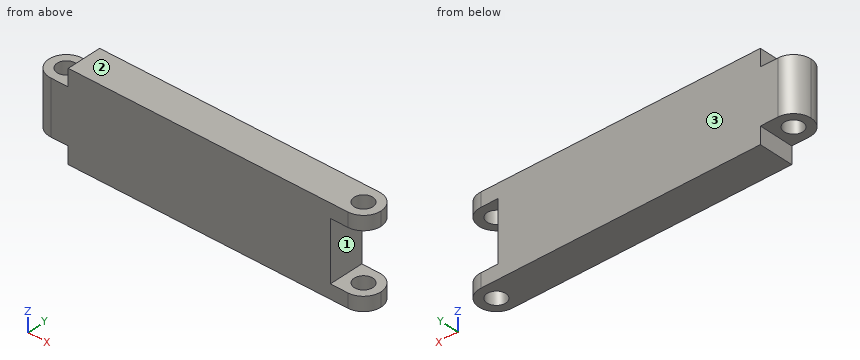
from build123d import *

# Parameters (mm, degrees)
SKETCH_1_W           = 57
SKETCH_1_H           = 15
EXTRUDE_5_DEPTH      = 6
SKETCH_13_W          = 6
SKETCH_13_H          = 10.2
CUT_EXTRUDE_8_DEPTH  = 6
SKETCH_14_R          = 1.6
CUT_EXTRUDE_9_DEPTH  = 17
SKETCH_15_W          = 6
SKETCH_15_H          = 2.4
CUT_EXTRUDE_10_DEPTH = 17
SKETCH_16_R          = 1.6
CUT_EXTRUDE_11_DEPTH = 17
SKETCH_17_W          = 6
SKETCH_17_H          = 6
CUT_EXTRUDE_12_DEPTH = 0.5
SKETCH_18_W          = 6
SKETCH_18_H          = 6
CUT_EXTRUDE_13_DEPTH = 0.5


with BuildPart() as part:
    # 草图1 → 凸台-拉伸5 (new body)
    with BuildSketch(Plane(origin=(0, 0, 0), x_dir=(1, 0, 0), z_dir=(0, 1, 0))):
        with Locations((5.252559727, 3.394197952)):
            Rectangle(SKETCH_1_W, SKETCH_1_H)
    extrude(amount=EXTRUDE_5_DEPTH)

    # 草图13 → 切除-拉伸8 (cut)
    with BuildSketch(Plane(origin=(0, 6, 0), x_dir=(1, 0, 0), z_dir=(0, 1, 0))):
        with Locations((30.752559727, 3.394197952)):
            Rectangle(SKETCH_13_W, SKETCH_13_H)
    extrude(amount=-CUT_EXTRUDE_8_DEPTH, mode=Mode.SUBTRACT)

    # 草图14 → 切除-拉伸9 (cut)
    with BuildSketch(Plane.XY.offset(4.105802048)):
        with Locations((30.752559727, 3)):
            Circle(SKETCH_14_R)
        with BuildLine():
            Line((33.752559727, 6), (30.752559727, 6))
            ThreePointArc((30.752559727, 6), (32.873880071, 5.121320344), (33.752559727, 3))
            Line((33.752559727, 3), (33.752559727, 6))
        make_face()
        with BuildLine():
            Line((33.752559727, 0), (33.752559727, 3))
            ThreePointArc((33.752559727, 3), (32.873880071, 0.878679656), (30.752559727, 0))
            Line((30.752559727, 0), (33.752559727, 0))
        make_face()
    extrude(amount=-CUT_EXTRUDE_9_DEPTH, mode=Mode.SUBTRACT)

    # 草图15 → 切除-拉伸10 (cut)
    with BuildSketch(Plane(origin=(0, 6, 0), x_dir=(1, 0, 0), z_dir=(0, 1, 0))):
        with Locations((-20.247440273, 9.694197952)):
            Rectangle(SKETCH_15_W, SKETCH_15_H)
        with Locations((-20.247440273, -2.905802048)):
            Rectangle(SKETCH_15_W, SKETCH_15_H)
    extrude(amount=-CUT_EXTRUDE_10_DEPTH, mode=Mode.SUBTRACT)

    # 草图16 → 切除-拉伸11 (cut)
    with BuildSketch(Plane.XY.offset(1.705802048)):
        with Locations((-20.247440273, 3)):
            Circle(SKETCH_16_R)
        with BuildLine():
            ThreePointArc((-23.247440273, 3), (-22.368760617, 5.121320344), (-20.247440273, 6))
            Line((-20.247440273, 6), (-23.247440273, 6))
            Line((-23.247440273, 6), (-23.247440273, 3))
        make_face()
        with BuildLine():
            ThreePointArc((-20.247440273, 0), (-22.368760617, 0.878679656), (-23.247440273, 3))
            Line((-23.247440273, 3), (-23.247440273, 0))
            Line((-23.247440273, 0), (-20.247440273, 0))
        make_face()
    extrude(amount=-CUT_EXTRUDE_11_DEPTH, mode=Mode.SUBTRACT)

    # 草图17 → 切除-拉伸12 (cut)
    with BuildSketch(Plane(origin=(0, 0, -8.494197952), x_dir=(-1, 0, 0), z_dir=(0, 0, -1))):
        with Locations((20.247440273, 3)):
            Rectangle(SKETCH_17_W, SKETCH_17_H)
    extrude(amount=-CUT_EXTRUDE_12_DEPTH, mode=Mode.SUBTRACT)

    # 草图18 → 切除-拉伸13 (cut)
    with BuildSketch(Plane.XY.offset(1.705802048)):
        with Locations((-20.247440273, 3)):
            Rectangle(SKETCH_18_W, SKETCH_18_H)
    extrude(amount=-CUT_EXTRUDE_13_DEPTH, mode=Mode.SUBTRACT)


solid = part.part
Can you work these out from the model? Positions are in its coordinate system, mm. Face numbers are marked on the shaded views. Round coordinates to 2 decimals unless told otherwise and drop trailing zeros. Order: outer loops, then holes, each group sorted by start corner. A loop starts at its lowest first (then second) coordinate and runs counter-clockwise, first axis right, second up. Notation, with made-up numbers: (72, 2) -> (131, 2) arc R21 ccw to (131, 40) -> close; hole circle Ø5 at (78.5, 43). An arc over 180 degrees is marked (long way). Write each question's results on one line, items separated by ' | '. Start each with the question number.
Item 1: Thinking about a two-plate mould opening in Z: for the marked faces 1, 2 and 3, which applies, +Z half, -Z half, draft (parallel to the pull), parting line (faces both ways), or undercut?
Item 2: If we section it at B-B, the plane y = 0.5: Write out the boundary of the cut face in (x, z), then the cut area to 3 significant figures.
Item 3: If we section it at A-A, the plane z = 2.5: Write out the boundary of the cut face in (x, y).
Item 4: If we section it at C-C, the plane y = 5.4: Write out the boundary of the cut face in (x, z), then the cut area to 3 significant figures.
Item 5: Please list where these lines run through material, in increasing order: L1, parallel to X at y = 3.05, z = -9; L2, parallel to X at y = 2.95, z = -3; L3, parallel to Z at x = 31, y = 5.3.
Item 6: Will these pins go through, and if not, where does the flat tip stop? pin 1 (3 mm diameter, centred on y = 1.5, z = -0.5, fed in from +X); pin 2 (2 mm diameter, centred on x = 25.5, z = -4.5, fed in from -Y); pin 3 (1.8 mm diameter, centred on x = -19, y = 3.5, fed in from -Z); pin 4 (1.4 mm diameter, centred on y = 4.5, z = -9.5, fed in from -X).
Results:
1) face 1: undercut | face 2: +Z half | face 3: draft
2) outline: (-21.91, -7.99) -> (-17.25, -7.99) -> (-17.25, -10.89) -> (32.41, -10.89) -> (32.41, -8.49) -> (27.75, -8.49) -> (27.75, 1.71) -> (32.41, 1.71) -> (32.41, 4.11) -> (-17.25, 4.11) -> (-17.25, 1.21) -> (-21.91, 1.21) -> close | area: 740 mm2
3) outline: (-17.25, 0) -> (30.75, 0) arc R3 ccw to (30.75, 6) -> (-17.25, 6) -> close; hole circle Ø3.2 at (30.75, 3)
4) outline: (-22.05, -7.99) -> (-17.25, -7.99) -> (-17.25, -10.89) -> (32.55, -10.89) -> (32.55, -8.49) -> (27.75, -8.49) -> (27.75, 1.71) -> (32.55, 1.71) -> (32.55, 4.11) -> (-17.25, 4.11) -> (-17.25, 1.21) -> (-22.05, 1.21) -> close | area: 742 mm2
5) L1: x = -17.25 to 29.15, 32.35 to 33.75 | L2: x = -23.25 to -21.85, -18.65 to 27.75 | L3: z = -10.89 to -8.49, 1.71 to 4.11
6) pin 1: stops at x = 27.75 | pin 2: stops at y = 0 | pin 3: stops at z = -7.99 | pin 4: stops at x = -17.25
